For this review, take the finished solid that the model builds, in its own axes (mm). Round coordinates to 2 decimals unless told otherwise and drop trailing zeros. Write each loop counter-clockwise with the first axis right and the second up, starting at its lowest first coordinate (ties: lowest second). Pieces come first, ordered by that corner, then holes. Notation, with made-up numbers: (5, 7.5) -> (37, 7.5) arc R18 cw to (37, 20.5) -> close; hole circle Ø11 at (42, 78.5). An arc over 180 degrees is marked (long way). Answer in a Markdown table with one row per item.
from build123d import *

# Parameters (mm, degrees)
Y_KSEKLIK_EKSTR_ZYON2_DEPTH = 10
IZIM3_W                     = 10
IZIM3_H                     = 40
Y_KSEKLIK_EKSTR_ZYON3_DEPTH = 10
IZIM4_W                     = 10
IZIM4_H                     = 104.5
Y_KSEKLIK_EKSTR_ZYON4_DEPTH = 10
IZIM6_W                     = 10
IZIM6_H                     = 50
Y_KSEKLIK_EKSTR_ZYON5_DEPTH = 10
IZIM7_W                     = 10
IZIM7_H                     = 94.5
Y_KSEKLIK_EKSTR_ZYON6_DEPTH = 10
IZIM8_R                     = 1.5
KES_EKSTR_ZYON1_DEPTH       = 35
IZIM9_R                     = 1.5
KES_EKSTR_ZYON2_DEPTH       = 265.5
IZIM12_R                    = 51
KES_EKSTR_ZYON4_DEPTH       = 338
Y_KSEKLIK_EKSTR_ZYON7_DEPTH = 5
Y_KSEKLIK_EKSTR_ZYON8_DEPTH = 5
IZIM21_W                    = 13.275114184
IZIM21_H                    = 150
KES_EKSTR_ZYON5_DEPTH       = 2.5
IZIM22_W                    = 15.470706389
IZIM22_H                    = 150
KES_EKSTR_ZYON6_DEPTH       = 2.5
IZIM23_R                    = 1.5
KES_EKSTR_ZYON7_DEPTH       = 242


with BuildPart() as part:
    # Çizim1 → Yükseklik-Ekstrüzyon2 (new body)
    with BuildSketch(Plane.XY):
        Polygon((-160, 54.142135624), (-104.644660941, 109.497474683), (104.644660941, 109.497474683), (160, 54.142135624), (160, -54.142135624), (104.644660941, -109.497474683), (-104.644660941, -109.497474683), (-160, -54.142135624), align=None)
        Polygon((-150, 50), (-150, -50), (-100.502525317, -99.497474683), (100.502525317, -99.497474683), (150, -50), (150, 50), (100.502525317, 99.497474683), (-100.502525317, 99.497474683), align=None, mode=Mode.SUBTRACT)
    extrude(amount=Y_KSEKLIK_EKSTR_ZYON2_DEPTH)

    # Çizim3 → Yükseklik-Ekstrüzyon3 (add)
    with BuildSketch(Plane(origin=(0, -104.5, 0), x_dir=(1, 0, 0), z_dir=(0, 1, 0))):
        with Locations((-99.644660941, -30)):
            Rectangle(IZIM3_W, IZIM3_H)
    y_kseklik_ekstr_zyon3 = extrude(amount=Y_KSEKLIK_EKSTR_ZYON3_DEPTH)

    # Çizim4 → Yükseklik-Ekstrüzyon4 (add)
    with BuildSketch(Plane.XY.offset(50)):
        with Locations((-99.644660941, -52.25)):
            Rectangle(IZIM4_W, IZIM4_H)
    y_kseklik_ekstr_zyon4 = extrude(amount=Y_KSEKLIK_EKSTR_ZYON4_DEPTH)

    # Çizim6 → Yükseklik-Ekstrüzyon5 (add)
    with BuildSketch(Plane(origin=(0, -94.5, 0), x_dir=(1, 0, 0), z_dir=(0, 1, 0))):
        with Locations((116.355339059, -35)):
            Rectangle(IZIM6_W, IZIM6_H)
    y_kseklik_ekstr_zyon5 = extrude(amount=Y_KSEKLIK_EKSTR_ZYON5_DEPTH)

    # Çizim7 → Yükseklik-Ekstrüzyon6 (add)
    with BuildSketch(Plane.XY.offset(50)):
        with Locations((116.355339059, -47.25)):
            Rectangle(IZIM7_W, IZIM7_H)
    y_kseklik_ekstr_zyon6 = extrude(amount=Y_KSEKLIK_EKSTR_ZYON6_DEPTH)

    # Aynalama1: Yükseklik-Ekstrüzyon3, Yükseklik-Ekstrüzyon4, Yükseklik-Ekstrüzyon5, Yükseklik-Ekstrüzyon6 across plane
    add(y_kseklik_ekstr_zyon3.mirror(Plane.ZX))
    add(y_kseklik_ekstr_zyon4.mirror(Plane.ZX))
    add(y_kseklik_ekstr_zyon5.mirror(Plane.ZX))
    add(y_kseklik_ekstr_zyon6.mirror(Plane.ZX))

    # Çizim8 → Kes-Ekstrüzyon1 (cut)
    with BuildSketch(Plane.XY.offset(10)):
        with Locations((145, 62.071067812)):
            Circle(IZIM8_R)
        with Locations((139.343145751, 67.727922061)):
            Circle(IZIM8_R)
        with Locations((139.343145751, -67.727922061)):
            Circle(IZIM8_R)
        with Locations((145, -62.071067812)):
            Circle(IZIM8_R)
        with Locations((-136.343145751, 70.727922061)):
            Circle(IZIM8_R)
        with Locations((-142, 65.071067812)):
            Circle(IZIM8_R)
        with Locations((-136.343145751, -70.727922061)):
            Circle(IZIM8_R)
        with Locations((-142, -65.071067812)):
            Circle(IZIM8_R)
        with Locations((-155, 0)):
            Circle(IZIM8_R)
    extrude(amount=-KES_EKSTR_ZYON1_DEPTH, mode=Mode.SUBTRACT)

    # Çizim9 → Kes-Ekstrüzyon2 (cut, symmetric)
    with BuildSketch(Plane(origin=(0, -94.5, 0), x_dir=(1, 0, 0), z_dir=(0, 1, 0))):
        with Locations(Location((-4, -4.992750184, 0), (0, 0, 90))):
            Circle(IZIM9_R)
        with Locations(Location((4, -4.992750184, 0), (0, 0, 90))):
            Circle(IZIM9_R)
    extrude(amount=KES_EKSTR_ZYON2_DEPTH, both=True, mode=Mode.SUBTRACT)

    # Çizim12 → Kes-Ekstrüzyon4 (cut, symmetric)
    with BuildSketch(Plane(origin=(-99.64, 0, 0), x_dir=(0, 0, -1), z_dir=(1, 0, 0))):
        with Locations((-69.443489697, 0)):
            Circle(IZIM12_R)
    extrude(amount=KES_EKSTR_ZYON4_DEPTH, both=True, mode=Mode.SUBTRACT)

    # Çizim19 → Yükseklik-Ekstrüzyon7 (add, symmetric)
    with BuildSketch(Plane(origin=(-99.64, 0, 0), x_dir=(0, 0, -1), z_dir=(1, 0, 0))):
        with BuildLine():
            Line((-50, -62.023791471), (-50, -47.148178209))
            ThreePointArc((-50, -47.148178209), (-18.443489697, 0), (-50, 47.148178209))
            Line((-50, 47.148178209), (-50, 62.023791471))
            ThreePointArc((-50, 62.023791471), (-4.443489697, 0), (-50, -62.023791471))
        make_face()
    extrude(amount=Y_KSEKLIK_EKSTR_ZYON7_DEPTH, both=True)

    # Çizim20 → Yükseklik-Ekstrüzyon8 (add, symmetric)
    with BuildSketch(Plane(origin=(116.36, 0, 0), x_dir=(0, 0, -1), z_dir=(1, 0, 0))):
        with BuildLine():
            Line((-50, -47.148178209), (-50, -62.023791471))
            ThreePointArc((-50, -62.023791471), (-4.443489697, 0), (-50, 62.023791471))
            Line((-50, 62.023791471), (-50, 47.148178209))
            ThreePointArc((-50, 47.148178209), (-18.443489697, 0), (-50, -47.148178209))
        make_face()
    extrude(amount=Y_KSEKLIK_EKSTR_ZYON8_DEPTH, both=True)

    # Çizim21 → Kes-Ekstrüzyon5 (cut, symmetric)
    with BuildSketch(Plane(origin=(-99.64, 0, 0), x_dir=(0, 0, -1), z_dir=(1, 0, 0))):
        with Locations((-56.637557092, 0)):
            Rectangle(IZIM21_W, IZIM21_H)
    extrude(amount=KES_EKSTR_ZYON5_DEPTH, both=True, mode=Mode.SUBTRACT)

    # Çizim22 → Kes-Ekstrüzyon6 (cut, symmetric)
    with BuildSketch(Plane(origin=(116.36, 0, 0), x_dir=(0, 0, -1), z_dir=(1, 0, 0))):
        with Locations((-57.735353195, 0)):
            Rectangle(IZIM22_W, IZIM22_H)
    extrude(amount=KES_EKSTR_ZYON6_DEPTH, both=True, mode=Mode.SUBTRACT)

    # Çizim23 → Kes-Ekstrüzyon7 (cut, symmetric)
    with BuildSketch(Plane(origin=(-99.64, 0, 0), x_dir=(0, 0, -1), z_dir=(1, 0, 0))):
        with Locations((-56.443489697, 60)):
            Circle(IZIM23_R)
        with Locations((-56.443489697, -60)):
            Circle(IZIM23_R)
    extrude(amount=KES_EKSTR_ZYON7_DEPTH, both=True, mode=Mode.SUBTRACT)


solid = part.part
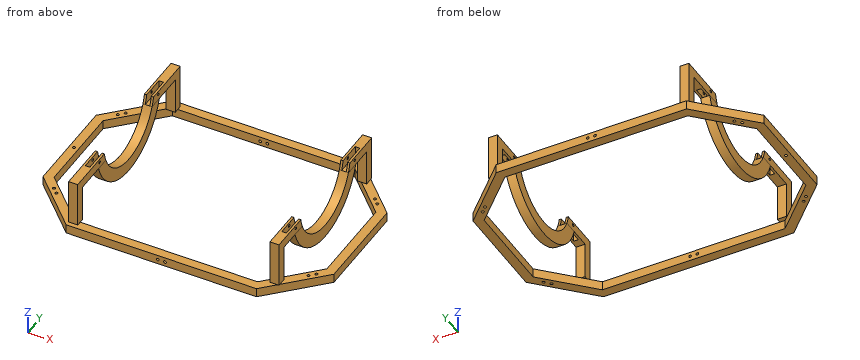
1) Consider section D-D on y = 43.5. State the section outline as (x, z) points.
Solved:
| item | result |
|---|---|
| outline | (-160, 0) -> (-150, 0) -> (-150, 10) -> (-160, 10) -> close; (-104.64, 21.14) -> (-94.64, 21.14) -> (-94.64, 42.82) -> (-104.64, 42.82) -> close; (111.36, 21.14) -> (121.36, 21.14) -> (121.36, 42.82) -> (111.36, 42.82) -> close; (150, 0) -> (160, 0) -> (160, 10) -> (150, 10) -> close |
2) Consider section A-A on x = -25.5. State the section outline as (y, z) points.
Solved:
| item | result |
|---|---|
| outline | (-109.5, 0) -> (-99.5, 0) -> (-99.5, 10) -> (-109.5, 10) -> close; (99.5, 0) -> (109.5, 0) -> (109.5, 10) -> (99.5, 10) -> close |
3) Clearance check with flat-ended pins moving along their axes: pin 1 Ø3 at (x, z) = (116, 43.5) entering from +Y; pin 2 Ø3.5 at (x, y) = (-136.34, 70.73) entering from +Z; pin 3 Ø11 at (y, z) = (-59.5, 54.5) entering from +X; pin 4 Ø10 at (y, z) = (2.5, 14) entering from -X. State where each tip first meets the part, or that it passes through.
Solved:
| item | result |
|---|---|
| pin 1 | y = 94.5 |
| pin 2 | z = 10 |
| pin 3 | x = 121.36 |
| pin 4 | x = -160 |
4) Consider section B-B on y = -11. State the section outline as (x, z) points.
Solved:
| item | result |
|---|---|
| outline | (-160, 0) -> (-150, 0) -> (-150, 10) -> (-160, 10) -> close; (-104.64, 5.38) -> (-94.64, 5.38) -> (-94.64, 19.64) -> (-104.64, 19.64) -> close; (111.36, 5.38) -> (121.36, 5.38) -> (121.36, 19.64) -> (111.36, 19.64) -> close; (150, 0) -> (160, 0) -> (160, 10) -> (150, 10) -> close |
5) Consider section C-C on z = 34. State how many separate pieces and enclosed holes the cut face has, then the cut area to 3 significant figures.
Solved:
| item | result |
|---|---|
| separate pieces | 8 |
| enclosed holes | 0 |
| area | 1,110 mm² |
6) For line 1 (Z direction, x = 4, y = 102.75); line 2 (X direction, y = 49.5, z = 31); line 3 (Y direction, x = -27.5, z = 9), list the stretches that pass through material, from the lowest coordinate up. Write a range as [from, to].
Solved:
| item | result |
|---|---|
| line 1 | [0, 3.49], [6.49, 10] |
| line 2 | [-104.64, -94.64], [111.36, 121.36] |
| line 3 | [-109.5, -99.5], [99.5, 109.5] |
